```python
from build123d import *

# Parameters (mm, degrees)
SKETCH1_W           = 100
SKETCH1_H           = 75
BOSS_EXTRUDE1_DEPTH = 45
SKETCH2_W           = 15
SKETCH2_H           = 25
CUT_EXTRUDE1_DEPTH  = 78.014609004
SKETCH3_W           = 30.197143083
SKETCH3_H           = 100
CUT_EXTRUDE2_DEPTH  = 78.014609004


with BuildPart() as part:
    # Sketch1 → Boss-Extrude1 (new body)
    with BuildSketch(Plane(origin=(0, 0, 0), x_dir=(0, 1, 0), z_dir=(0, 0, 1))):
        Rectangle(SKETCH1_W, SKETCH1_H)
    extrude(amount=BOSS_EXTRUDE1_DEPTH)

    # Sketch2 → Cut-Extrude1 (cut, through all)
    with BuildSketch(Plane.XY.offset(45)):
        Polygon((-15.5, 18), (-32.5, 18), (-32.5, -45), (32.5, -45), (32.5, 45), (-15.5, 45), (-15.5, 20), align=None)
        with Locations((-25, 32.5)):
            Rectangle(SKETCH2_W, SKETCH2_H)
    extrude(amount=-CUT_EXTRUDE1_DEPTH, mode=Mode.SUBTRACT)

    # Sketch3 → Cut-Extrude2 (cut, through all)
    with BuildSketch(Plane.XY.offset(45)):
        with Locations((-0.401428459, 0)):
            Rectangle(SKETCH3_W, SKETCH3_H)
    extrude(amount=-CUT_EXTRUDE2_DEPTH, mode=Mode.SUBTRACT)


with BuildPart() as body_2:
    # of the pieces the cut leaves, the one that is kept (cut_extrude2_keep)
    add(part.part.solids().sort_by_distance((37.5, -50, 0))[0])


solid = body_2.part
```
Design review of the part built by this model. Coordinates are the model's own, in mm. A direction names the side the tool comes from. Give positions to 0.01 mm unless a question says otherwise; leave off trailing zeros. Loops run counter-clockwise (first coordinate to the right, second up) from the corner with the lowest first, then second, coordinate; pieces in that order, holes last. Notation, with made-up numbers: M -30.5,-33.75 L -12.5,-33.75 A21 cw -12.5,-19.75 Z; hole C -28,-39 d2. An arc over 180 degrees is marked long. Return JSON: item names as keys, results as strings. Group by question number.
Item 1: Insertion check: pin 1 Ø13.5 at (y, z) = (20, 28.5) entering from -X; pin 2 Ø2 at (x, y) = (30.5, -19.5) entering from -Z. Each pin has a flat end and moves straight along its axis. Give the tip position at first contact, or say it passes through.
Item 2: We need section B-B (z = 39). Give the boundary of the cut face in (x, y), and give its area (3 significant figures).
Item 3: Tool access review of faces 5 (the flat face through (32.5, -1, 23)), 6 (the flat face through (14.697, -48, 23)): name each direction out of +Z, -Z, +X, -X, +Y, -Y from which nothing blocks a thin tool from reaching the whole face with its end or side.
Item 4: We need section C-C (y = -7). Give the boundary of the cut face in (x, z).
Item 5: We need section A-A (x = 23.25). Give the boundary of the cut face in (y, z), and give its area (3 significant figures).
Item 6: Mouldability with a two-part tool opening along Y and no side actions: class faces 1 (the flat face through (23, -45, 23)), 2 (the flat face through (33, 0, 0)), 3 (the flat face through (24, 45, 23)), 4 (the flat face through (26, -50, 22)) as released by +Y, released by -Y, zero draft, split by the parting line, or undercut.
Item 7: For probe 1 along Y at (x, z) = (27.5, 31.5); probe 2 along X at (y, z) = (13, 7.5), list the stretches that pass through material, from the lowest coordinate up.
Output:
{
 "1": {"pin 1": "stops at x = 32.5", "pin 2": "passes through"},
 "2": {"outline": "M 14.7,-50 L 37.5,-50 L 37.5,50 L 14.7,50 L 14.7,45 L 32.5,45 L 32.5,-45 L 14.7,-45 Z", "area": "678 mm^2"},
 "3": {"face 5": "+Z, -Z, -X", "face 6": "+Z, -Z, -X, +Y, -Y"},
 "4": {"outline": "M 32.5,0 L 37.5,0 L 37.5,45 L 32.5,45 Z"},
 "5": {"outline": "M -50,0 L -45,0 L -45,45 L -50,45 Z; M 45,0 L 50,0 L 50,45 L 45,45 Z", "area": "450 mm^2"},
 "6": {"face 1": "undercut", "face 2": "zero draft", "face 3": "undercut", "face 4": "released by -Y"},
 "7": {"probe 1": "y = -50 to -45, 45 to 50", "probe 2": "x = 32.5 to 37.5"}
}
